Autodesk Inventor part; units mm, degrees
ref_plane "YZ Plane" through (0, 0, 0) normal (1, 0, 0) x (0, 1, 0)
ref_plane "XZ Plane" through (0, 0, 0) normal (0, 1, 0) x (-1, 0, 0)
ref_plane "XY Plane" through (0, 0, 0) normal (0, 0, 1) x (1, 0, 0)
ref_plane "Arbeitsebene1" through (0, 0, 50) normal (0, 0, 1) x (1, 0, 0)
sketch "Skizze1" plane through (0, 0, 50) normal (0, 0, 1) x (1, 0, 0)
  circle A0 centre (0, -2) radius 0.75
  line L0 (32.5, 30.5) -> (-32.5, 30.5)
  line L1 (-32.5, 30.5) -> (-32.5, -34.5)
  line L2 (-32.5, -34.5) -> (32.5, -34.5)
  line L3 (32.5, -34.5) -> (32.5, 30.5)
  line L4 (32.5, 30.5) -> (-32.5, -34.5) construction
  line L5 (-32.5, 30.5) -> (32.5, -34.5) construction
  point P0 (0, 0)
  dimension "d0" = 65
  dimension "d1" = 65
extrude "Extrusion1" add sketch "Skizze1" along normal blind 1
sketch "Skizze2" plane through (0, 0, 50) normal (0, 0, 1) x (1, 0, 0)
  circle A0 centre (0, -2) radius 0.75
  line L0 (32.5, 30.5) -> (-32.5, 30.5)
  line L1 (-32.5, 30.5) -> (-32.5, -34.5)
  line L2 (-32.5, -34.5) -> (32.5, -34.5)
  line L3 (32.5, -34.5) -> (32.5, 30.5)
  circle A1 centre (0, -33.1) radius 1
  circle A2 centre (0, 29.1) radius 1
  circle A3 centre (8.2, -33.1) radius 1
  circle A4 centre (-8.2, -33.1) radius 1
  circle A5 centre (-8.2, 29.1) radius 1
  circle A6 centre (8.2, 29.1) radius 1
  point P0 (0, 0)
  point P1 (3.8, 10.2517)
  dimension "d4" = 2
  dimension "d5" = 2
  dimension "d6" = 1.4
  dimension "d7" = 1.4
  dimension "d8" = 2
  dimension "d9" = 2
  dimension "d10" = 2
  dimension "d11" = 2
extrude "Extrusion2" cut sketch "Skizze2" along normal blind 1 contours A1 | A2 | A3 | A4 | A5 | A6
pattern_circular "Runde Anordnung1" count 4 over 360 about axis through (0, -2, 50) along (0, 0, 1) of "Extrusion2"
properties part number "00_LED-ARRAY"
Model file for the job. Use its own axes, mm. Give positions to 0.01 mm unless a question says otherwise; leave off trailing zeros. Loops run counter-clockwise (first coordinate to the right, second up) from the corner with the lowest first, then second, coordinate; pieces in that order, holes last. Notation, with made-up numbers: (10.25, -34) -> (18.25, -34) arc R19 cw to (18.25, -21) -> close; hole circle Ø1 at (42.5, 61). An arc over 180 degrees is marked (long way). Use a Markdown table: item, result. Add a question column.
(1) Slice it at C-C on y = -10.2. List the corners of the cut face in (x, z), and give its area (3 significant figures).
(2) Slice it at B-B on x = 8.2. List the corners of the cut face in (y, z), and give its area (3 significant figures).
(3) Wall check: line 1 along X through (y, z) = (-10.2, 50.75); line 2 along Y through (x, z) = (31.1, 50.4); line 3 along Y through (x, z) = (0, 50.8). Give the ranges that are in metal, low to high.
(4) Mould opens along X. For faces 1 (the cylindrical face through (-8.33, 28.11, 50.49)), 2 (the cylindrical face through (-0.13, 28.11, 50.49)), 3 (the flat face through (-8, -2, 50)) say: +X half, -X half, draft (parallel to the pull), parting line (faces both ways), or undercut.
(5) Slice it at D-D on y = -2. List the corners of the cut face in (x, z).
(6) Slice it at A-A on y = -33.1. List the corners of the cut face in (x, z), and give its area (3 significant figures).
Filled sheet:
| question | item | result |
|---|---|---|
| 1 | outline | (-32.5, 50) -> (-32.1, 50) -> (-32.1, 51) -> (-32.5, 51) -> close; (-30.1, 50) -> (30.1, 50) -> (30.1, 51) -> (-30.1, 51) -> close; (32.1, 50) -> (32.5, 50) -> (32.5, 51) -> (32.1, 51) -> close |
| 1 | area | 61.0 mm2 |
| 2 | outline | (-34.5, 50) -> (-34.1, 50) -> (-34.1, 51) -> (-34.5, 51) -> close; (-32.1, 50) -> (28.1, 50) -> (28.1, 51) -> (-32.1, 51) -> close; (30.1, 50) -> (30.5, 50) -> (30.5, 51) -> (30.1, 51) -> close |
| 2 | area | 61.0 mm2 |
| 3 | line 1 | -32.5 to -32.1, -30.1 to 30.1, 32.1 to 32.5 |
| 3 | line 2 | -34.5 to -11.2, -9.2 to -3, -1 to 5.2, 7.2 to 30.5 |
| 3 | line 3 | -34.5 to -34.1, -32.1 to -2.75, -1.25 to 28.1, 30.1 to 30.5 |
| 4 | face 1 | undercut |
| 4 | face 2 | undercut |
| 4 | face 3 | draft |
| 5 | outline | (-32.5, 50) -> (-32.1, 50) -> (-32.1, 51) -> (-32.5, 51) -> close; (-30.1, 50) -> (-0.75, 50) -> (-0.75, 51) -> (-30.1, 51) -> close; (0.75, 50) -> (30.1, 50) -> (30.1, 51) -> (0.75, 51) -> close; (32.1, 50) -> (32.5, 50) -> (32.5, 51) -> (32.1, 51) -> close |
| 6 | outline | (-32.5, 50) -> (-9.2, 50) -> (-9.2, 51) -> (-32.5, 51) -> close; (-7.2, 50) -> (-1, 50) -> (-1, 51) -> (-7.2, 51) -> close; (1, 50) -> (7.2, 50) -> (7.2, 51) -> (1, 51) -> close; (9.2, 50) -> (32.5, 50) -> (32.5, 51) -> (9.2, 51) -> close |
| 6 | area | 59.0 mm2 |
